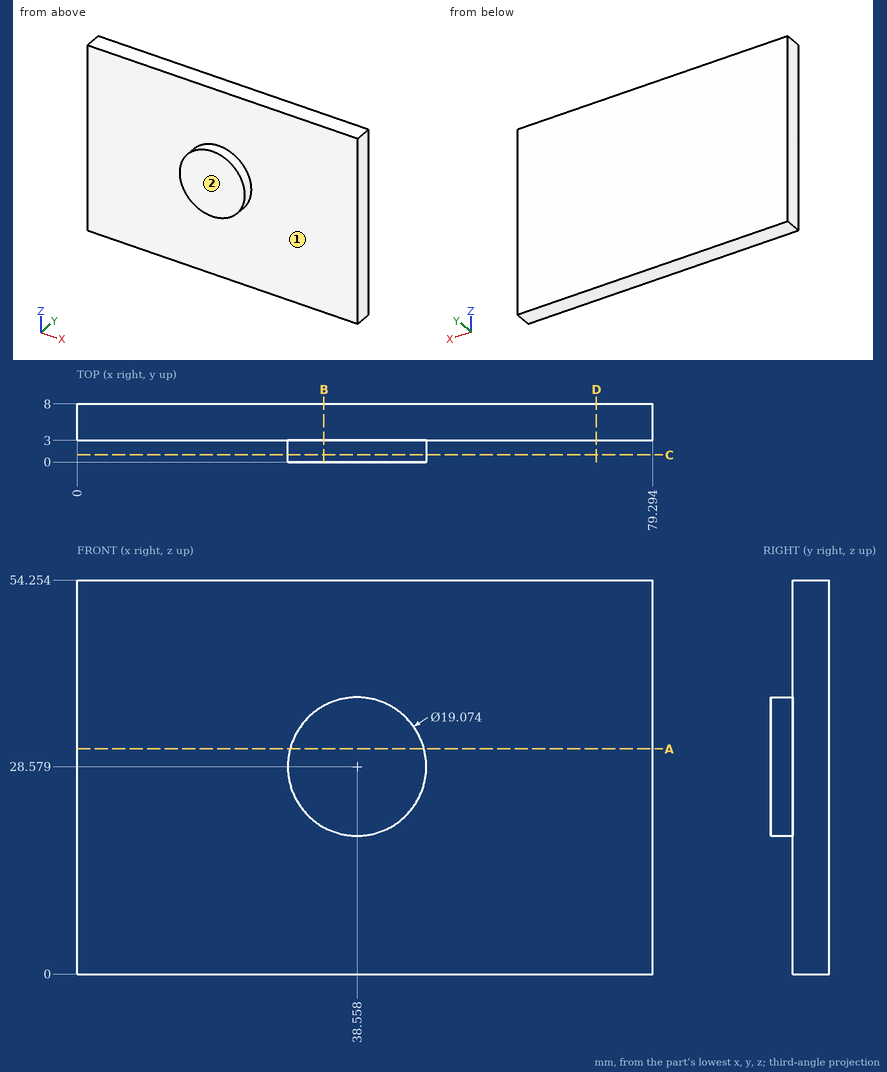
Geometry check sheet. Reference: drawing and pictorial views, mm from the part's lowest x, y, z. A direction names the side the tool comes from. Coordinates: 2 decimals unless noted, no trailing zeros. Write each loop counter-clockwise with the first axis right and the second up, starting at its lowest first coordinate (ties: lowest second). Pieces come first, ordered by that corner, then holes. Notation, with made-up numbers: M 16,-18.5 L 33,-18.5 A26 ccw 33,16.5 Z; hole C 69.25,71.5 d1. An arc over 180 degrees is marked long. Write item = value, one per line. Start each with the question number.
1. Sectioned sample at C-C (y = 1). Record the cut outline in (x, z) (1 decimal), then the cut area to 3 significant figures.
2. Go/stop test with a flat-tipped pin: pin 1 (8 mm diameter, centred on x = 59, z = 13, fed in from -Y). Record where the tip stops, or that it passes through.
3. Tool access check on the marked faces 1 and 2. Record the directions out of +Z, -Z, +X, -X, +Y, -Y that give a thin tool (end or side, any length) a straight path to the whole face; none if there is none.
4. Sectioned sample at B-B (x = 34). Record the cut outline in (y, z) (1 decimal).
5. Sectioned sample at D-D (x = 71.5). Record the cut outline in (y, z).
6. Thickness scan on probe 1 along Y at (x, z) = (6, 51); probe 2 along Z at (x, y) = (45, 2) (1 decimal); probe 3 along Z at (x, y) = (46, 2.75) (1 decimal). Record the ranges inside material, lowest first.
7. Sectioned sample at A-A (z = 31). Record the cut outline in (x, y), then the cut area to 3 significant figures.
The answers:
q1.outline = C 38.6,28.6 d19.1
q1.area = 286 mm²
q2.pin_1 = 3
q3.face_1 = -Y
q3.face_2 = +Z, -Z, +X, -X, -Y
q4.outline = M 0,20.2 L 3,20.2 L 3,0 L 8,0 L 8,54.3 L 3,54.3 L 3,37 L 0,37 Z
q5.outline = M 3,0 L 8,0 L 8,54.25 L 3,54.25 Z
q6.probe_1 = 3 to 8
q6.probe_2 = 21.5 to 35.6
q6.probe_3 = 22.6 to 34.5
q7.outline = M 0,3 L 29.33,3 L 29.33,0 L 47.78,0 L 47.78,3 L 79.29,3 L 79.29,8 L 0,8 Z
q7.area = 452 mm²
